Geometry check sheet. Reference: the model listing, model coordinates, mm. Face numbers are marked on the shaded views. Give positions to 0.01 mm unless a question says otherwise; leave off trailing zeros. Write each loop counter-clockwise with the first axis right and the second up, starting at its lowest first coordinate (ties: lowest second). Pieces come first, ordered by that corner, then holes. Notation, with made-up numbers: (64.25, -23) - (102.25, -23) arc R31 ccw to (102.25, 11) - close; hole circle Ø7 at (-13, -0.75). An arc over 180 degrees is marked (long way). One line per question, with ' | ' between items. Start each with the question number.
Q1. Section check A-A on y = 0. Record the boundary of the cut face in (x, z).
Q2. Section check D-D on x = -33. Record the boundary of the cut face in (y, z), and give its area (3 significant figures).
Q3. Thickness scan on L1, parallel to Y at x = 0, z = 19.5; L2, parallel to Z at x = 19, y = -15; L3, parallel to X at y = 21.5, z = 31. Record the ranges inside material, lowest first. Write a range as [from, to].
Q4. Section check B-B on x = 0. Record the boundary of the cut face in (y, z).
Q5. Gauge pin test, flat ends, axial feed: P1, Ø3, axis at y = 36.5, z = 29.5, coming from the -X side; P2, Ø8, axis at x = -17.5, z = 43, coming from the +Y side; P3, Ø6, axis at x = 7, z = 28.5, coming from the -Y side. Record the tip position at first contact, or that the pin passes through.
Q6. Release check for a two-part mould opening along X. For the marked faces 1, 2 and 3 record: +X half, -X half, draft (parallel to the pull), parting line (faces both ways), or undercut.
Q7. Section check C-C on z = 26. Record the boundary of the cut face in (x, y).
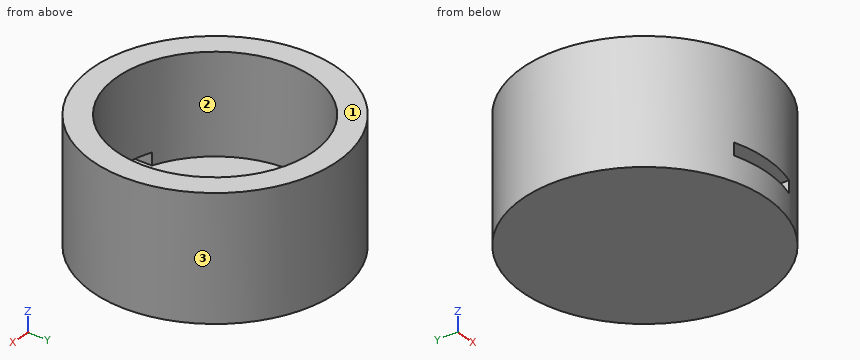
```python
from build123d import *

# Parameters (mm, degrees)
SKETCH1_R           = 50
BOSS_EXTRUDE1_DEPTH = 50
SKETCH2_R           = 40
CUT_EXTRUDE1_DEPTH  = 40
SKETCH3_W           = 30
SKETCH3_H           = 5
CUT_EXTRUDE2_DEPTH  = 193


with BuildPart() as part:
    # Sketch1 → Boss-Extrude1 (new body)
    with BuildSketch(Plane.XY):
        Circle(SKETCH1_R)
    extrude(amount=BOSS_EXTRUDE1_DEPTH)

    # Sketch2 → Cut-Extrude1 (cut)
    with BuildSketch(Plane.XY.offset(50)):
        Circle(SKETCH2_R)
    extrude(amount=-CUT_EXTRUDE1_DEPTH, mode=Mode.SUBTRACT)

    # Sketch3 → Cut-Extrude2 (cut)
    with BuildSketch(Plane(origin=(0, 0, 0), x_dir=(1, 0, 0), z_dir=(0, 1, 0))):
        with Locations((0, -12.5)):
            Rectangle(SKETCH3_W, SKETCH3_H)
    extrude(amount=-CUT_EXTRUDE2_DEPTH, mode=Mode.SUBTRACT)


solid = part.part
```
Working result:
1) outline: (-50, 0) - (50, 0) - (50, 50) - (40, 50) - (40, 10) - (-40, 10) - (-40, 50) - (-50, 50) - close
2) outline: (-37.56, 0) - (37.56, 0) - (37.56, 50) - (22.61, 50) - (22.61, 10) - (-22.61, 10) - (-22.61, 50) - (-37.56, 50) - close | area: 1,950 mm2
3) L1: y = [-50, -40], [40, 50] | L2: z = [0, 10] | L3: x = [-45.14, -33.73], [33.73, 45.14]
4) outline: (-50, 0) - (50, 0) - (50, 50) - (40, 50) - (40, 10) - (-50, 10) - close; (-50, 15) - (-40, 15) - (-40, 50) - (-50, 50) - close
5) P1: stops at x = -35.71 | P2: stops at y = 48.14 | P3: stops at y = -49.84
6) face 1: draft | face 2: undercut | face 3: parting line
7) outline: circle Ø100 at (0, 0); hole circle Ø80 at (0, 0)
